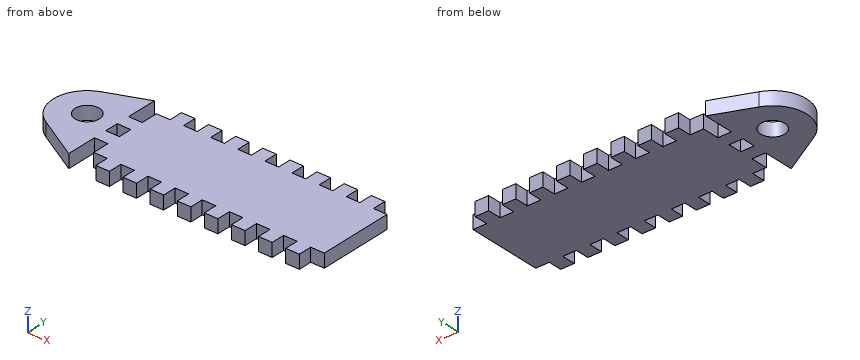
```python
from build123d import *

# Parameters (mm, degrees)
MASS_DEPTH          = 6.35
SKETCH4_R           = 5.715
CUT_EXTRUDE1_DEPTH  = 102.024858757
SKETCH3_W           = 6.35
SKETCH3_H           = 12.7
CUT_EXTRUDE2_DEPTH  = 102.024858757
CAVITY1_START       = -14.457315323
CAVITY1_OUTLINE_W   = 6.35
CAVITY1_OUTLINE_H   = 6.35
CAVITY1_DEPTH       = 14.2875
CAVITY1_START_2     = 18.880184677
CAVITY1_2_OUTLINE_W = 6.35
CAVITY1_2_OUTLINE_H = 6.35
CAVITY1_2_DEPTH     = 14.2875
CAVITY1_START_3     = 6.180184677
CAVITY1_3_OUTLINE_W = 6.35
CAVITY1_3_OUTLINE_H = 6.35
CAVITY1_3_DEPTH     = 6.35
LPATTERN1_COUNT     = 9
LPATTERN1_PITCH     = 12.7


# Read off the part's stored shape, not the designer's step: Cavity1
with BuildPart() as part:
    # Sketch1 → Mass (new body)
    with BuildSketch(Plane.XY):
        with BuildLine():
            Line((-19.086533096, -14.457315323), (95.213466904, -14.457315323))
            Line((95.213466904, -14.457315323), (95.213466904, 33.167684677))
            Line((95.213466904, 33.167684677), (-19.086533096, 33.167684677))
            Line((-19.086533096, 33.167684677), (-37.714474787, 25.669365644))
            ThreePointArc((-37.714474787, 25.669365644), (-47.627354737, 11.983835347), (-39.590998194, -2.881422872))
            Line((-39.590998194, -2.881422872), (-19.086533096, -14.457315323))
        make_face()
    extrude(amount=MASS_DEPTH)

    # Sketch4 → Cut-Extrude1 (cut, through all)
    with BuildSketch(Plane(origin=(0, 0, 0), x_dir=(-1, 0, 0), z_dir=(0, 0, -1))):
        with Locations((31.786533096, 10.942684677)):
            Circle(SKETCH4_R)
    extrude(amount=-CUT_EXTRUDE1_DEPTH, mode=Mode.SUBTRACT)

    # Sketch3 → Cut-Extrude2 (cut, through all)
    with BuildSketch(Plane(origin=(0, 0, 0), x_dir=(-1, 0, 0), z_dir=(0, 0, -1))):
        with Locations((-92.038466904, 33.164228805)):
            Rectangle(SKETCH3_W, SKETCH3_H)
        with Locations((-92.038466904, -14.457315323)):
            Rectangle(SKETCH3_W, SKETCH3_H)
    cut_extrude2 = extrude(amount=-CUT_EXTRUDE2_DEPTH, mode=Mode.SUBTRACT)

    # Cavity1 outline → Cavity1 (cut)
    with BuildSketch(Plane(origin=(0, 0, 0), x_dir=(1, 0, 0), z_dir=(0, 1, 0)).offset(CAVITY1_START)):
        with Locations((-15.911533096, -3.175)):
            Rectangle(CAVITY1_OUTLINE_W, CAVITY1_OUTLINE_H)
    extrude(amount=CAVITY1_DEPTH, mode=Mode.SUBTRACT)

    # Cavity1 2 outline → Cavity1 2 (cut)
    with BuildSketch(Plane(origin=(0, 0, 0), x_dir=(1, 0, 0), z_dir=(0, 1, 0)).offset(CAVITY1_START_2)):
        with Locations((-15.911533096, -3.175)):
            Rectangle(CAVITY1_2_OUTLINE_W, CAVITY1_2_OUTLINE_H)
    extrude(amount=CAVITY1_2_DEPTH, mode=Mode.SUBTRACT)

    # Cavity1 3 outline → Cavity1 3 (cut)
    with BuildSketch(Plane(origin=(0, 0, 0), x_dir=(1, 0, 0), z_dir=(0, 1, 0)).offset(CAVITY1_START_3)):
        with Locations((-15.911533096, -3.175)):
            Rectangle(CAVITY1_3_OUTLINE_W, CAVITY1_3_OUTLINE_H)
    extrude(amount=CAVITY1_3_DEPTH, mode=Mode.SUBTRACT)

    # LPattern1: Cut-Extrude2 ×9
    with Locations(*[(-i * LPATTERN1_PITCH, 0, 0) for i in range(1, LPATTERN1_COUNT)]):
        add(cut_extrude2, mode=Mode.SUBTRACT)


solid = part.part
```
Here's how the part is built. I have some questions about the finished solid (model axes, mm). Coordinates: 2 decimals unless noted, no trailing zeros. Write each loop counter-clockwise with the first axis right and the second up, starting at its lowest first coordinate (ties: lowest second). Pieces come first, ordered by that corner, then holes. Notation, with made-up numbers: M 24.5,-10 L 79.5,-10 A28 ccw 79.5,14 Z; hole C 13.25,33.5 d9. An arc over 180 degrees is marked long. Answer as CSV lines item,"result". Start each with the question number.
Q1. Will these pins go through, and if not, where does the flat tip stop? pin 1 Ø1.5 at (x, y) = (76.5, 2.5) entering from -Z; pin 2 Ø1.9 at (y, z) = (-12.5, 4) entering from +X; pin 3 Ø1.9 at (y, z) = (-12, 4) entering from -X; pin 4 Ø1.9 at (x, z) = (-17, 3) entering from -Y.
Q2. I need wall thicknesses on probe 1 along X at (y, z) = (12.5, 1.5); probe 2 along X at (y, z) = (10, 5); probe 3 along X at (y, z) = (25, 1.25). Which ranges of each line are inside material? Lowest first, please. Write a range as [from, to].
Q3. Suppose I cut it at B-B, the plane x = -36. List the corners of the cut face in (y, z) for me, then the cut area to 3 significant figures.
Q4. Suppose I cut it at A-A, the plane x = -16. List the corners of the cut face in (y, z) for me, then the cut area to 3 significant figures.
Q5. Suppose I cut it at C-C, the plane y = 29.5. State how many separate pieces and enclosed holes the cut face has, then the cut area to 3 significant figures.
Entries:
1,pin 1,"stops at z = 0"
1,pin 2,"stops at x = 88.86"
1,pin 3,"stops at x = -25.12"
1,pin 4,"stops at y = -0.17"
2,probe 1,"x = [-47.58, -37.29], [-26.29, -19.09], [-12.74, 95.21]"
2,probe 2,"x = [-47.63, -37.42], [-26.15, -19.09], [-12.74, 95.21]"
2,probe 3,"x = [-39.16, -19.09], [-12.74, 95.21]"
3,outline,"M -4.91,0 L 7.08,0 L 7.08,6.35 L -4.91,6.35 Z; M 14.8,0 L 26.36,0 L 26.36,6.35 L 14.8,6.35 Z"
3,area,"150 mm²"
4,outline,"M -0.17,0 L 6.18,0 L 6.18,6.35 L -0.17,6.35 Z; M 12.53,0 L 18.88,0 L 18.88,6.35 L 12.53,6.35 Z"
4,area,"80.6 mm²"
5,separate pieces,"9"
5,enclosed holes,"0"
5,area,"380 mm²"
